```python
from build123d import *

# Parameters (mm, degrees)
F0_W     = 13
F0_H     = 13
F1_DEPTH = 3
F2_R     = 1
F3_DEPTH = 4
F4_R     = 1
F5_DEPTH = 4


with BuildPart() as f1:
    # F0 (on Top) → F1 (new body)
    with BuildSketch(Plane.XY):
        with Locations((6.5, 6.5)):
            Rectangle(F0_W, F0_H)
    extrude(amount=F1_DEPTH)

    # F2 (on face) → F3 (join)
    with BuildSketch(Plane.XZ):
        with Locations((1.5, 1.5)):
            Circle(F2_R)
        with Locations((11.5, 1.5)):
            Circle(F2_R)
    extrude(amount=F3_DEPTH)

    # F4 (on face) → F5 (join)
    with BuildSketch(Plane(origin=(0, 13, 0), x_dir=(-1, 0, 0), z_dir=(0, 1, 0))):
        with Locations((-11.5, 1.5)):
            Circle(F4_R)
        with Locations((-1.5, 1.5)):
            Circle(F4_R)
    extrude(amount=F5_DEPTH)


solid = f1.part
```
Geometry: final body of the model. Coordinates: model frame, mm. A direction names the side the tool comes from. Round coordinates to 2 decimals unless told otherwise and drop trailing zeros. Order: outer loops, then holes, each group sorted by start corner. A loop starts at its lowest first (then second) coordinate and runs counter-clockwise, first axis right, second up. Notation, with made-up numbers: (42, 42) - (86, 42) arc R29 cw to (86, 70) - close; hole circle Ø6 at (81.25, 87). An arc over 180 degrees is marked (long way). Use CSV: the item, a comma, the result in double quotes. Start each with the question number.
Q1. Section query D-D (x = 8.5). Return loops of the section in (y, z), and give its area (3 significant figures).
Q2. Mould query, pull axis X, two halves, no side actions, for faces 4 (the face through (12, 17, 2)), 5 (the face through (12.3, 15, 0.9)), 6 (the face through (0, 6, 1)). Classes: +X half, -X half, draft (parallel to the pull), parting line (faces both ways), or undercut.
Q3. Section query C-C (x = 11). Return loops of the section in (y, z), and give its area (3 significant figures).
Q4. Access query for faces 1 (the face through (6, 0, 1)), 2 (the face through (2, 17, 2)), 3 (the face through (1.717, 14.972, 0.524)). Directions: +Z, -Z, +X, -X, +Y, -Y. A direction counts if a zero-diameter tool reaches every point of the face in a straight line with its end or side. Return the directions, or none.
Q5. Section query A-A (z = 1.5). Return loops of the section in (x, y).
Q6. Section query B-B (x = 1.5). Return loops of the section in (y, z).
Q7. Material intervals for line 1 along Y through (x, z) = (6.25, 0.65); line 2 along X through (y, z) = (-2.5, 2); line 3 along X through (y, z) = (-2.5, 1.75), sorted ascending. Write a range as from..to.
Result set:
1,outline,"(0, 0) - (13, 0) - (13, 3) - (0, 3) - close"
1,area,"39.0 mm2"
2,face 4,"draft"
2,face 5,"undercut"
2,face 6,"-X half"
3,outline,"(-4, 0.63) - (0, 0.63) - (0, 0) - (13, 0) - (13, 0.63) - (17, 0.63) - (17, 2.37) - (13, 2.37) - (13, 3) - (0, 3) - (0, 2.37) - (-4, 2.37) - close"
3,area,"52.9 mm2"
4,face 1,"-Y"
4,face 2,"+Z, -Z, +X, -X, +Y"
4,face 3,"+Y"
5,outline,"(0, 0) - (0.5, 0) - (0.5, -4) - (2.5, -4) - (2.5, 0) - (10.5, 0) - (10.5, -4) - (12.5, -4) - (12.5, 0) - (13, 0) - (13, 13) - (12.5, 13) - (12.5, 17) - (10.5, 17) - (10.5, 13) - (2.5, 13) - (2.5, 17) - (0.5, 17) - (0.5, 13) - (0, 13) - close"
6,outline,"(-4, 0.5) - (0, 0.5) - (0, 0) - (13, 0) - (13, 0.5) - (17, 0.5) - (17, 2.5) - (13, 2.5) - (13, 3) - (0, 3) - (0, 2.5) - (-4, 2.5) - close"
7,line 1,"y = 0..13"
7,line 2,"x = 0.63..2.37, 10.63..12.37"
7,line 3,"x = 0.53..2.47, 10.53..12.47"
